```python
from build123d import *

# Parameters (mm, degrees)
BOSS_EXTRUDE1_DEPTH = 6.35
CUT_EXTRUDE1_DEPTH  = 6.35


with BuildPart() as part:
    # Sketch1 → Boss-Extrude1 (new body)
    with BuildSketch(Plane.XY):
        Polygon((76.2, 190.5), (76.2, 203.2), (69.85, 203.2), (69.85, 304.8), (76.2, 304.8), (76.2, 317.5), (69.85, 317.5), (69.85, 444.5), (76.2, 444.5), (76.2, 457.2), (69.85, 457.2), (69.85, 508), (6.35, 508), (6.35, 457.2), (0, 457.2), (0, 444.5), (6.35, 444.5), (6.35, 317.5), (0, 317.5), (0, 304.8), (6.35, 304.8), (6.35, 203.2), (0, 203.2), (0, 190.5), (6.35, 190.5), (6.35, 63.5), (0, 63.5), (0, 50.8), (6.35, 50.8), (6.35, 6.35), (69.85, 6.35), (69.85, 50.8), (76.2, 50.8), (76.2, 63.5), (69.85, 63.5), (69.85, 190.5), align=None)
    extrude(amount=BOSS_EXTRUDE1_DEPTH)

    # Sketch2 → Cut-Extrude1 (cut)
    with BuildSketch(Plane(origin=(0, 0, 0), x_dir=(-1, 0, 0), z_dir=(0, 0, -1))):
        Polygon((-58.7375, 124.61875), (-55.5625, 124.61875), (-55.5625, 129.38125), (-58.7375, 129.38125), (-58.7375, 131.7625), (-61.9125, 131.7625), (-61.9125, 129.38125), (-69.85, 129.38125), (-69.85, 124.61875), (-61.9125, 124.61875), (-61.9125, 122.2375), (-58.7375, 122.2375), align=None)
        Polygon((-6.35, 124.61875), (-14.2875, 124.61875), (-14.2875, 122.2375), (-17.4625, 122.2375), (-17.4625, 124.61875), (-20.6375, 124.61875), (-20.6375, 129.38125), (-17.4625, 129.38125), (-17.4625, 131.7625), (-14.2875, 131.7625), (-14.2875, 129.38125), (-6.35, 129.38125), align=None)
        Polygon((-17.4625, 383.38125), (-20.6375, 383.38125), (-20.6375, 378.61875), (-17.4625, 378.61875), (-17.4625, 376.2375), (-14.2875, 376.2375), (-14.2875, 378.61875), (-6.35, 378.61875), (-6.35, 383.38125), (-14.2875, 383.38125), (-14.2875, 385.7625), (-17.4625, 385.7625), align=None)
        Polygon((-69.85, 383.38125), (-61.9125, 383.38125), (-61.9125, 385.7625), (-58.7375, 385.7625), (-58.7375, 383.38125), (-55.5625, 383.38125), (-55.5625, 378.61875), (-58.7375, 378.61875), (-58.7375, 376.2375), (-61.9125, 376.2375), (-61.9125, 378.61875), (-69.85, 378.61875), align=None)
    extrude(amount=-CUT_EXTRUDE1_DEPTH, mode=Mode.SUBTRACT)


solid = part.part
```
Part model, mm, in its own coordinate system. Coordinates: 2 decimals unless noted, no trailing zeros. Write each loop counter-clockwise with the first axis right and the second up, starting at its lowest first coordinate (ties: lowest second). Pieces come first, ordered by that corner, then holes.
Item 1: Slice it at A-A (y = 391.5). Write the cut outline in (x, z).
Item 2: Probe line 1 (Y direction, x = 61, z = 3.75); line 2 (Y direction, x = 71, z = 1); line 3 (Y direction, x = 18.5, z = 6). List the from-to ranges inside material, lowest first.
Item 3: Pin check, flat tips, straight feed: pin 1 (1.9 mm diameter, centred on x = 72.5, z = 2.5, fed in from +Y); pin 2 (1.9 mm diameter, centred on y = 148.5, z = 4.5, fed in from -X); pin 3 (1.9 mm diameter, centred on y = 377.5, z = 2, fed in from +X); pin 4 (10 mm diameter, centred on x = 10.5, y = 174.5, fed in from -Z). Stop position of each tip, or through.
Results found:
1. outline: (6.35, 0) - (69.85, 0) - (69.85, 6.35) - (6.35, 6.35) - close
2. line 1: y = 6.35 to 122.24, 131.76 to 376.24, 385.76 to 508
2. line 2: y = 50.8 to 63.5, 190.5 to 203.2, 304.8 to 317.5, 444.5 to 457.2
2. line 3: y = 6.35 to 124.62, 129.38 to 378.62, 383.38 to 508
3. pin 1: stops at y = 457.2
3. pin 2: stops at x = 6.35
3. pin 3: stops at x = 69.85
3. pin 4: stops at z = 0
